```python
from build123d import *

# Parameters (mm, degrees)
SKETCH_W          = 30.48
SKETCH_H          = 125
SKETCH_R          = 1.6
PAD_DEPTH         = 4.064
SKETCH001_W       = 30.48
SKETCH001_H       = 30.48
SKETCH001_R       = 1.6
PAD001_DEPTH      = 4
FILLET_R          = 2.286
PAD002_DEPTH      = 5
SKETCH003_W       = 4
SKETCH003_H       = 3
SKETCH003_W_2     = 10
PAD003_DEPTH      = 2
PAD004_DEPTH      = 15.24
PAD004_DEPTH_BACK = 15.24
SKETCH005_R       = 9.5
POCKET_DEPTH      = 5
SKETCH006_W       = 8
SKETCH006_H       = 3
PAD005_DEPTH      = 2
SKETCH007_W       = 6
SKETCH007_H       = 7
POCKET001_DEPTH   = 10


with BuildPart() as part:
    # Sketch → Pad (new body)
    with BuildSketch(Plane.XZ):
        with Locations((0, 62.5)):
            Rectangle(SKETCH_W, SKETCH_H)
        with Locations((-8.89, 69.28)):
            Circle(SKETCH_R, mode=Mode.SUBTRACT)
        with Locations((8.89, 69.28)):
            Circle(SKETCH_R, mode=Mode.SUBTRACT)
        with Locations((-8.89, 115)):
            Circle(SKETCH_R, mode=Mode.SUBTRACT)
        with Locations((8.89, 115)):
            Circle(SKETCH_R, mode=Mode.SUBTRACT)
        with Locations((-3.81, 29.21)):
            Circle(SKETCH_R, mode=Mode.SUBTRACT)
        with Locations((8.89, 29.21)):
            Circle(SKETCH_R, mode=Mode.SUBTRACT)
        with Locations((-3.81, 8.89)):
            Circle(SKETCH_R, mode=Mode.SUBTRACT)
        with Locations((8.89, 8.89)):
            Circle(SKETCH_R, mode=Mode.SUBTRACT)
    extrude(amount=-PAD_DEPTH)

    # Sketch001 → Pad001 (join)
    with BuildSketch(Plane.XY):
        with Locations((0, -15.24)):
            Rectangle(SKETCH001_W, SKETCH001_H)
        with Locations((0, -5.08)):
            Circle(SKETCH001_R, mode=Mode.SUBTRACT)
        with Locations((0, -25.4)):
            Circle(SKETCH001_R, mode=Mode.SUBTRACT)
        with Locations((10.16, -15.24)):
            Circle(SKETCH001_R, mode=Mode.SUBTRACT)
        with Locations((-10.16, -15.24)):
            Circle(SKETCH001_R, mode=Mode.SUBTRACT)
    extrude(amount=PAD001_DEPTH)

    # Fillet
    fillet_edges = [part.edges().sort_by_distance(p)[0] for p in [
        (0, 0, 4),
    ]]
    fillet(fillet_edges, radius=FILLET_R)

    # Sketch002 (on Face6 of Pad001) → Pad002 (join)
    with BuildSketch(Plane(origin=(0, 0, 125), x_dir=(-1, 0, 0), z_dir=(0, 0, 1))):
        with BuildLine():
            Line((-15.24, 30.48), (-15.24, 0))
            Line((-15.24, 0), (-6, 0))
            Line((-6, 0), (-6, 12.13454))
            ThreePointArc((6, 12.13454), (0, 29), (-6, 12.13454))
            Line((6, 12.13454), (6, 0))
            Line((6, 0), (15.24, 0))
            Line((15.24, 0), (15.24, 30.48))
            Line((15.24, 30.48), (-15.24, 30.48))
        make_face()
    extrude(amount=-PAD002_DEPTH)

    # Sketch003 (on Face3 of Pad002) → Pad003 (join)
    with BuildSketch(Plane.XZ):
        with Locations((0, 69.28)):
            Rectangle(SKETCH003_W, SKETCH003_H)
        with Locations((0, 115)):
            Rectangle(SKETCH003_W_2, SKETCH003_H)
    extrude(amount=PAD003_DEPTH)

    # Sketch004 → Pad004 (join, two sides)
    with BuildSketch(Plane.YZ) as pad004_sk:
        Polygon((0, 47.68), (-3.5, 47.68), (-11.040195, 60.74), (-30.48, 60.74), (-30.48, 46.87), (0, 33.81), align=None)
    extrude(amount=PAD004_DEPTH)
    extrude(pad004_sk.sketch, amount=-PAD004_DEPTH_BACK)

    # Sketch005 (on Face30 of Pad004) → Pocket (cut)
    with BuildSketch(Plane(origin=(0, 0, 60.74), x_dir=(-1, 0, 0), z_dir=(0, 0, 1))):
        with Locations((0, 19.5)):
            Circle(SKETCH005_R)
    extrude(amount=-POCKET_DEPTH, mode=Mode.SUBTRACT)

    # Sketch006 (on Face5 of Pocket) → Pad005 (join)
    with BuildSketch(Plane.XZ):
        with Locations((2.54, 29.21)):
            Rectangle(SKETCH006_W, SKETCH006_H)
        with Locations((2.54, 8.89)):
            Rectangle(SKETCH006_W, SKETCH006_H)
    extrude(amount=PAD005_DEPTH)

    # Sketch007 (on Face16 of Pad005) → Pocket001 (cut)
    with BuildSketch(Plane(origin=(0, 0, 47.68), x_dir=(-1, 0, 0), z_dir=(0, 0, 1))):
        with Locations((7.24, 3.5)):
            Rectangle(SKETCH007_W, SKETCH007_H)
    extrude(amount=POCKET001_DEPTH, mode=Mode.SUBTRACT)


solid = part.part
```
Could you check a few things on this model? Use its own coordinates, in mm. A direction names the side the tool comes from. Round coordinates to 2 decimals unless told otherwise and drop trailing zeros. Loops run counter-clockwise (first coordinate to the right, second up) from the corner with the lowest first, then second, coordinate; pieces in that order, holes last. Notation, with made-up numbers: M -11,34.5 L 31,34.5 A25 cw 31,67.5 Z; hole C 59,78.25 d8. An arc over 180 degrees is marked long. Write item = value, one per line.
1. I need wall thicknesses on probe 1 along X at (y, z) = (2.55, 115); probe 2 along Z at (x, y) = (8, 2); probe 3 along Z at (x, y) = (-11.5, -11.5). Which ranges of each line are inside material? Lowest first, please.
Results below:
probe_1 = -15.24 to -10.49, -7.29 to 7.29, 10.49 to 15.24
probe_2 = 0 to 7.56, 10.22 to 27.88, 30.54 to 67.95, 70.61 to 113.67, 116.33 to 125
probe_3 = 0 to 4, 38.74 to 60.74, 120 to 125
2. Which directions (+Z, -Z, +X, -X, +Y, -Y) give clear straight access to the entire face, cutting with the end or side of a thin tool? Please do faces 4 (the face through (2, -1, 7.39)), 5 (the face through (0, -29, 123)), 6 (the face through (-1.46, -1, 9)), 7 (the face through (-10.24, -6, 49)), 8 (the face through (5, -1, 115)).
Results below:
face_4 = +X, -X, -Y
face_5 = +Z
face_6 = -X, -Y
face_7 = none
face_8 = +Z, +X, -Y
3. I want a section at D-D, the plane y = -5.08. Write out the boundary of the cut face in (x, z), and give its area (3 significant figures).
Results below:
outline = M -15.24,0 L -1.6,0 L -1.6,4 L -15.24,4 Z; M -15.24,35.99 L 15.24,35.99 L 15.24,50.42 L -4.24,50.42 L -4.24,47.68 L -10.24,47.68 L -10.24,50.42 L -15.24,50.42 Z; M -15.24,120 L -6,120 L -6,125 L -15.24,125 Z; M 1.6,0 L 15.24,0 L 15.24,4 L 1.6,4 Z; M 6,120 L 15.24,120 L 15.24,125 L 6,125 Z
area = 625 mm²
4. Will these pins go through, and if not, where does the flat tip stop? P1, Ø6, axis at x = 4, z = 23.5, coming from the -Y side; P2, Ø0.6, axis at y = -1.5, z = 29.5, coming from the -X side; P3, Ø0.6, axis at x = 2.5, y = -1, coming from the +Z side; P4, Ø1.9, axis at x = 8.89, z = 69.28, coming from the +Y side.
Results below:
P1 = 0
P2 = -1.46
P3 = 116.5
P4 = through
5. I want a section at A-A, the plane z = 115. Write out the boundary of the cut face in (x, y).
Results below:
outline = M -15.24,0 L -10.49,0 L -10.49,4.06 L -15.24,4.06 Z; M -7.29,0 L -5,0 L -5,-2 L 5,-2 L 5,0 L 7.29,0 L 7.29,4.06 L -7.29,4.06 Z; M 10.49,0 L 15.24,0 L 15.24,4.06 L 10.49,4.06 Z
6. I want a section at B-B, the plane y = -19.5. Write out the boundary of the cut face in (x, z), and give its area (3 significant figures).
Results below:
outline = M -15.24,0 L 15.24,0 L 15.24,4 L -15.24,4 Z; M -15.24,42.17 L 15.24,42.17 L 15.24,60.74 L 9.5,60.74 L 9.5,55.74 L -9.5,55.74 L -9.5,60.74 L -15.24,60.74 Z; M -15.24,120 L -9.5,120 L -9.5,125 L -15.24,125 Z; M 9.5,120 L 15.24,120 L 15.24,125 L 9.5,125 Z
area = 650 mm²
7. Thinking about a two-plate mould opening in Y: for faces 1 (the face through (-2, -1, 69)), 2 (the face through (0, 4.064, 63)), 3 (the face through (6, -6, 123)), which applies, +Y half, -Y half, draft (parallel to the pull), parting line (faces both ways), or undercut?
Results below:
face_1 = draft
face_2 = +Y half
face_3 = undercut
8. I want a section at C-C, the plane z = 69.28. Write out the boundary of the cut face in (x, y).
Results below:
outline = M -15.24,0 L -10.49,0 L -10.49,4.06 L -15.24,4.06 Z; M -7.29,0 L -2,0 L -2,-2 L 2,-2 L 2,0 L 7.29,0 L 7.29,4.06 L -7.29,4.06 Z; M 10.49,0 L 15.24,0 L 15.24,4.06 L 10.49,4.06 Z
